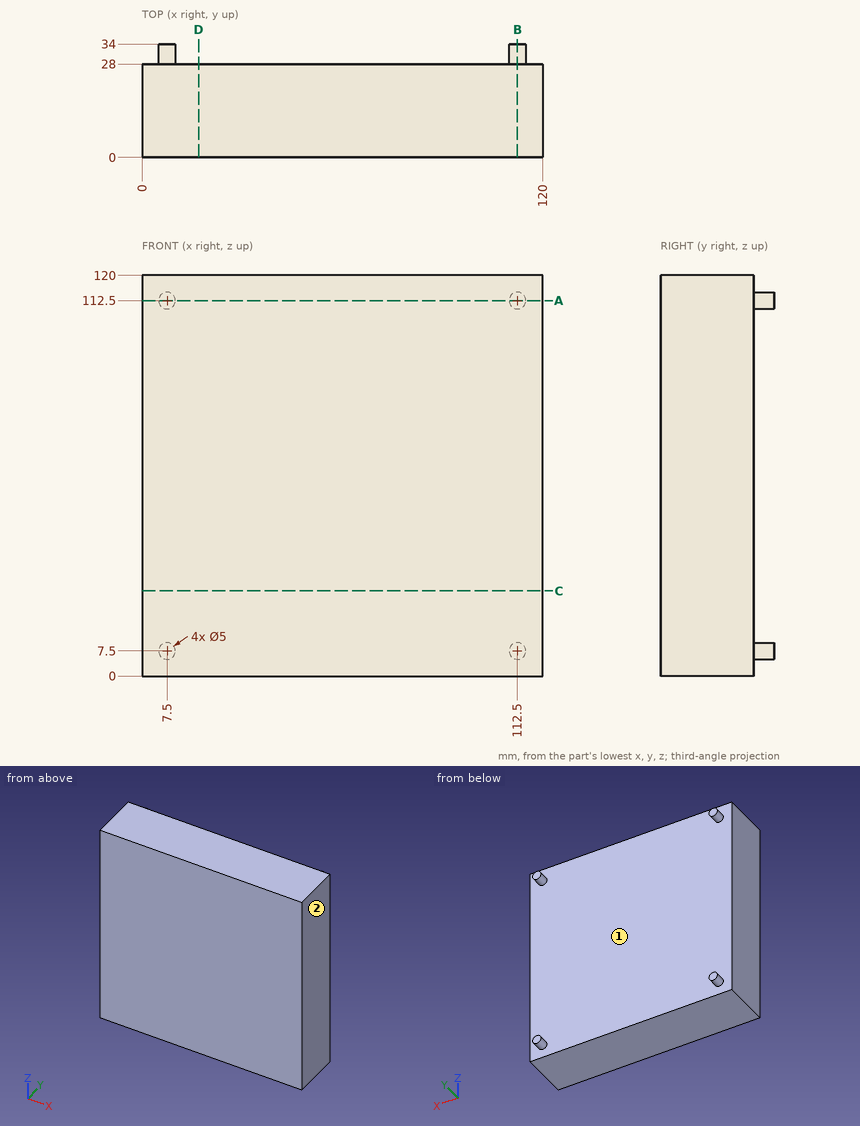
Study the drawing (mm; zero at the part's minimum x, y, z) and answer. A direction names the side the tool comes from. Give positions to 0.01 mm unless a question says otherwise; leave off trailing zeros. Loops run counter-clockwise (first coordinate to the right, second up) from the corner with the lowest first, then second, coordinate; pieces in that order, holes last. Notation, with made-up numbers: (19, 13.5) - (74, 13.5) arc R20 ccw to (74, 24.5) - close; hole circle Ø5 at (33, 86.25). An arc over 180 degrees is marked (long way). Answer as CSV lines item,"result". Start each with the question number.
1) Find section D-D (x = 17). Write down the section's boundary in (y, z), then the cut area to 3 significant figures.
2) Which of the six approach directions +Z, -Z, +X, -X, +Y, -Y give full straight-line access (tool end or side, diameter ignored) to the marked faces 1 and 2?
3) Find section C-C (z = 25.5). Write down the section's boundary in (x, y), then the cut area to 3 significant figures.
4) A straight line is drawn through the part: L1, parallel to Y at x = 31, z = 66.5. Find the intervals that lie inside material, in ascending order. Write a range as from..to.
5) This flat-tipped pin is pushed along its axis until it touches: pin 1 Ø1.5 at (x, z) = (28.5, 106.5) entering from +Y. Where does it stop, or does it pass through?
6) Find section A-A (z = 112.5). Write down the section's boundary in (x, y), then the cut area to 3 significant figures.
7) Find section B-B (x = 112.5). Write down the section's boundary in (y, z).
Findings below:
1,outline,"(0, 0) - (28, 0) - (28, 120) - (0, 120) - close"
1,area,"3,360 mm^2"
2,face 1,"+Y"
2,face 2,"+Z, -Z, +X, +Y, -Y"
3,outline,"(0, 0) - (120, 0) - (120, 28) - (0, 28) - close"
3,area,"3,360 mm^2"
4,L1,"0..28"
5,pin 1,"y = 28"
6,outline,"(0, 0) - (120, 0) - (120, 28) - (115, 28) - (115, 34) - (110, 34) - (110, 28) - (10, 28) - (10, 34) - (5, 34) - (5, 28) - (0, 28) - close"
6,area,"3,420 mm^2"
7,outline,"(0, 0) - (28, 0) - (28, 5) - (34, 5) - (34, 10) - (28, 10) - (28, 110) - (34, 110) - (34, 115) - (28, 115) - (28, 120) - (0, 120) - close"
